Could you check a few things on this model? Use its own coordinates, in mm. A direction names the side the tool comes from. Give positions to 0.01 mm unless a question says otherwise; leave off trailing zeros. Write each loop counter-clockwise with the first axis right and the second up, starting at its lowest first coordinate (ties: lowest second). Pieces come first, ordered by that corner, then holes. Notation, with made-up numbers: M 78,31 L 135,31 A35 ccw 135,68 Z; hole C -16,53 d11. An arc over 180 degrees is marked long. One line per item, written item: value.
```python
from build123d import *

# Parameters (mm, degrees)
F0_R     = 15
F1_DEPTH = 1
F2_R     = 16.075
F3_DEPTH = 3.5
F4_DEPTH = 1.5
F5_R     = 1.9
F6_DEPTH = 9.1


with BuildPart() as f1:
    # F0 (on Front) → F1 (new body)
    with BuildSketch(Plane.XZ):
        with BuildLine():
            Line((5, -26.5), (5, -16.77051))
            ThreePointArc((5, -16.77051), (0, 17.5), (-5, -16.77051))
            Line((-5, -16.77051), (-5, -26.5))
            Line((-5, -26.5), (5, -26.5))
        make_face()
        Circle(F0_R, mode=Mode.SUBTRACT)
    extrude(amount=F1_DEPTH)

    # F2 (on face) → F3 (join)
    with BuildSketch(Plane.XZ.offset(1)):
        with BuildLine():
            ThreePointArc((5, -16.77051), (14.031215, -10.45825), (17.5, 0))
            ThreePointArc((17.5, 0), (-10.45825, 14.031215), (-5, -16.77051))
            ThreePointArc((-5, -16.77051), (0, -17.5), (5, -16.77051))
        make_face()
        Circle(F2_R, mode=Mode.SUBTRACT)
    extrude(amount=F3_DEPTH)

    # F3_face (on face) → F4 (join)
    with BuildSketch(Plane(origin=(0, -1, -21.876907), x_dir=(1, 0, 0), z_dir=(0, -1, 0))):
        with BuildLine():
            ThreePointArc((5, 5.106397), (0, 4.376907), (-5, 5.106397))
            Line((-5, 5.106397), (-5, -4.623093))
            Line((-5, -4.623093), (5, -4.623093))
            Line((5, -4.623093), (5, 5.106397))
        make_face()
    extrude(amount=F4_DEPTH)

    # F5 (on face) → F6 (join)
    with BuildSketch(Plane.XZ.offset(2.5)):
        with Locations((0, -22.6)):
            Circle(F5_R)
    extrude(amount=F6_DEPTH)


solid = f1.part
```
1) We'd pull the mould along Z, two halves only. Please class faces 4 (the face through (0, -2.5, -20)), 5 (the face through (0, -1, -26.5)), 6 (the face through (5.1, -4.5, -15.5)): pulls with the +Z half, pulls with the -Z half, needs draft (parallel to the pull), parting line crosses it, or undercut.
Outcome:
face 4: undercut
face 5: pulls with the -Z half
face 6: needs draft
2) If we section it at D-D, the plane x = 7: Write out the boundary of the cut face in (y, z), then the cut area to 3 significant figures.
Outcome:
outline: M -4.5,-16.04 L 0,-16.04 L 0,-13.27 L -1,-13.27 L -1,-14.47 L -4.5,-14.47 Z; M -4.5,14.47 L -1,14.47 L -1,13.27 L 0,13.27 L 0,16.04 L -4.5,16.04 Z
area: 16.5 mm^2
3) On a 3-axis mill with a long thin cutter (end or side, diameter ignored), from which of +Z, -Z, +X, -X, +Y, -Y can I reach the whole of each face in a straight line? I mean faces 1 (the face through (-5, -1, -22)), 2 (the face through (11, -1, -11)), 3 (the face through (5, -1, -22)). Say none if no direction works.
Outcome:
face 1: -Z, -X, +Y, -Y
face 2: -Y
face 3: -Z, +X, +Y, -Y
4) I'm going to push flat-ended pins straight in: pin 1 (1.2 mm diameter, centred on y = -1.5, z = -21, fed in from -X); pin 2 (1.5 mm diameter, centred on x = -1, y = -10, fed in from -Z); pin 3 (10 mm diameter, centred on x = 10, z = 7.5, fed in from -Y). Where does each tip first touch, or does it pass through?
Outcome:
pin 1: stops at x = -5
pin 2: stops at z = -24.48
pin 3: stops at y = -4.5
5) If we section it at C-C, the plane z = -4: Write out the boundary of the cut face in (x, y).
Outcome:
outline: M -17.04,-4.5 L -15.57,-4.5 L -15.57,-1 L -14.46,-1 L -14.46,0 L -17.04,0 Z; M 14.46,-1 L 15.57,-1 L 15.57,-4.5 L 17.04,-4.5 L 17.04,0 L 14.46,0 Z
6) If we section it at A-A, the plane x = 0: Write out the boundary of the cut face in (y, z) (3 decimals), then the cut area to 3 significant figures.
Outcome:
outline: M -11.6,-24.5 L -2.5,-24.5 L -2.5,-26.5 L 0,-26.5 L 0,-15 L -1,-15 L -1,-16.075 L -4.5,-16.075 L -4.5,-17.5 L -2.5,-17.5 L -2.5,-20.7 L -11.6,-20.7 Z; M -4.5,16.075 L -1,16.075 L -1,15 L 0,15 L 0,17.5 L -4.5,17.5 Z
area: 72.1 mm^2
7) If we section it at B-B, the plane y = -3.5: Write out the boundary of the cut face in (x, z) (3 decimals).
Outcome:
outline: M -5,-16.771 A17.5 ccw 5,-16.771 A17.5 ccw 17.5,0 A17.5 ccw long Z; C 0,-22.6 d3.8; hole C 0,0 d32.15
8) Please list where these lines run through material, in increasing order: L1, parallel to Z at x = 0, y = -0.45; L2, parallel to Z at x = 0, y = -2.25 (3 decimals); L3, parallel to X at y = -1.5, z = -5. Write a range as from..to.
Outcome:
L1: z = -26.5..-15, 15..17.5
L2: z = -26.5..-16.075, 16.075..17.5
L3: x = -16.77..-15.28, 15.28..16.77
